Build history of the part. All positions in model axes, mm. A direction names the side the tool comes from. Coordinates: 2 decimals unless noted, no trailing zeros. Order: outer loops, then holes, each group sorted by start corner. A loop starts at its lowest first (then second) coordinate and runs counter-clockwise, first axis right, second up. Notation, with made-up numbers: (79.5, 21) - (94.5, 21) arc R27 cw to (94.5, 53) - close; hole circle Ø5 at (22, -16.5). An arc over 180 degrees is marked (long way). Write each question's results on one line, items separated by ' | '. Start each with the question number.
from build123d import *

# Parameters (mm, degrees)
EXTRUDE_1_DEPTH          = 105
SKETCH_7_W               = 30.4
SKETCH_7_H               = 19
EXTRUDE_2_DEPTH          = 3
SKETCH_8_W               = 30.4
SKETCH_8_H               = 12
EXTRUDE_3_DEPTH          = 38
FILLET_1_R               = 5
CUT_EXTRUDE_1_DEPTH      = 117
CUT_EXTRUDE_2_DEPTH      = 97
CUT_EXTRUDE_4_DEPTH      = 191.002631561
CUT_EXTRUDE_4_DEPTH_BACK = 6.8
SKETCH_11_R              = 5
FILLET_3_R               = 3
SKETCH_12_R              = 2.6
CUT_EXTRUDE_5_DEPTH      = 20
CHAMFER_1_SIZE           = 3
SKETCH_13_R              = 2.9
CUT_EXTRUDE_6_DEPTH      = 191.002631561
CHAMFER_3_SIZE           = 2.5
SKETCH_16_W              = 80
SKETCH_16_H              = 48
CUT_EXTRUDE_9_DEPTH      = 191.002631561
FILLET_4_R               = 30
SKETCH_17_W              = 28
SKETCH_17_H              = 52
CUT_EXTRUDE_10_DEPTH     = 20
FILLET_5_R               = 8
SKETCH_18_W              = 8
SKETCH_18_H              = 24
EXTRUDE_4_DEPTH          = 49
CHAMFER_4_SIZE           = 50
FILLET_6_R               = 10
SKETCH_19_R              = 2.9
CUT_EXTRUDE_11_DEPTH     = 191.002631561
CHAMFER_5_SIZE           = 2.6
SKETCH_21_R              = 2.3
CUT_EXTRUDE_13_DEPTH     = 15
FILLET_7_R               = 5
CHAMFER_6_SIZE           = 0.8
SKETCH_22_W              = 8
SKETCH_22_H              = 48.683816014
EXTRUDE_5_DEPTH          = 10
FILLET_8_R               = 10


with BuildPart() as part:
    # Sketch 2 → Extrude 1 (new body)
    with BuildSketch(Plane(origin=(0, 0, 0), x_dir=(1, 0, 0), z_dir=(0, 1, 0))):
        Polygon((52.378939236, 0), (52.378939236, -108), (24.378939236, -122), (24.378939236, -140), (0, -140), (-21.621060764, -140), (-21.621060764, 0), (-8.021060764, 0), (-8.021060764, -136), (0, -136), (22.378939236, -136), (22.378939236, 0), align=None)
    extrude(amount=EXTRUDE_1_DEPTH)



with BuildPart() as body_2:
    # Sketch 7 → Extrude 2 (new body)
    with BuildSketch(Plane.XZ):
        with Locations((7.178939236, 126.5)):
            Rectangle(SKETCH_7_W, SKETCH_7_H)
    extrude(amount=-EXTRUDE_2_DEPTH)


with BuildPart() as part_1:
    add(part.part)

    add(body_2.part)  # Extrude 3 merges body 2
    # Sketch 8 → Extrude 3 (add)
    with BuildSketch(Plane(origin=(0, 3, 0), x_dir=(1, 0, 0), z_dir=(0, 1, 0))):
        with Locations((7.178939236, -130)):
            Rectangle(SKETCH_8_W, SKETCH_8_H)
    extrude(amount=EXTRUDE_3_DEPTH)

    # Fillet 1
    fillet_1_edges = [part_1.edges().sort_by_distance(p)[0] for p in [
        (7.178939236, 41, 124),
    ]]
    fillet(fillet_1_edges, radius=FILLET_1_R)

    # Sketch 3 → Cut-Extrude 1 (cut)
    with BuildSketch(Plane(origin=(0, 0, 0), x_dir=(-1, 0, 0), z_dir=(0, 0, -1))):
        Polygon((8.021060764, -1.66), (19.321060764, 3.4), (19.321060764, 5), (8.021060764, 5), align=None)
        Polygon((-33.678939236, 5), (-22.378939236, 5), (-22.378939236, -1.66), (-33.678939236, 3.4), align=None)
    extrude(amount=-CUT_EXTRUDE_1_DEPTH, mode=Mode.SUBTRACT)

    # Sketch 9 → Cut-Extrude 2 (cut)
    with BuildSketch(Plane(origin=(0, 105, 0), x_dir=(1, 0, 0), z_dir=(0, 1, 0))):
        Polygon((-21.621060764, 0), (-21.621060764, -96), (22.378939236, -96), (22.378939236, -117), (47.378939236, -104.5), (47.378939236, 0), align=None)
    extrude(amount=-CUT_EXTRUDE_2_DEPTH, mode=Mode.SUBTRACT)

    # Sketch 11 → Cut-Extrude 4 (cut, two sides: drawn at the far end of the back side and taken through both)
    with BuildSketch(Plane.ZY.offset(21.621060764).offset(-CUT_EXTRUDE_4_DEPTH_BACK)):
        with Locations(Location((103.6, 41.2, 0), (0, 0, 180))):
            Circle(SKETCH_11_R)
    extrude(amount=CUT_EXTRUDE_4_DEPTH + CUT_EXTRUDE_4_DEPTH_BACK, mode=Mode.SUBTRACT)

    # Fillet 3
    fillet_3_edges = [part_1.edges().sort_by_distance(p)[0] for p in [
        (47.378939236, 56.5, 104.5),
        (22.378939236, 56.5, 117),
        (24.378939236, 52.5, 140),
        (24.378939236, 52.5, 122),
    ]]
    fillet(fillet_3_edges, radius=FILLET_3_R)

    # Sketch 12 → Cut-Extrude 5 (cut)
    with BuildSketch(Plane.ZY.offset(21.621060764)):
        with Locations((103.6, 41.2)):
            Circle(SKETCH_12_R)
    extrude(amount=-CUT_EXTRUDE_5_DEPTH, mode=Mode.SUBTRACT)

    # Chamfer 1
    # the kernel refuses this chamfer: 3 mm, written as the material it takes off along each edge
    with BuildSketch(Plane(origin=(-14.821060764, 41.2, 103.6), x_dir=(0, 0, 1), z_dir=(0, -1, 0))) as chamfer_1_piece_1_section:
        Polygon((2.6, -CHAMFER_1_SIZE), (2.6 + CHAMFER_1_SIZE, 0), (2.6, 0), align=None)
    chamfer_1_piece_1 = revolve(axis=Axis((-14.821060764, 41.2, 103.6), (-1, 0, 0)), mode=Mode.PRIVATE)
    chamfer_1_piece_1 = chamfer_1_piece_1 & Plane(origin=(-13.01179882, 41.2, 103.6), x_dir=(0, 0, -1), z_dir=(-1, 0, 0)) * Cylinder(5, 23, mode=Mode.PRIVATE)
    add(chamfer_1_piece_1, mode=Mode.SUBTRACT)

    # Sketch 13 → Cut-Extrude 6 (cut, through all)
    with BuildSketch(Plane.ZY.offset(21.621060764)):
        with Locations((88, 46)):
            Circle(SKETCH_13_R)
        with Locations((8, 46)):
            Circle(SKETCH_13_R)
        with Locations((88, 96)):
            Circle(SKETCH_13_R)
    extrude(amount=-CUT_EXTRUDE_6_DEPTH, mode=Mode.SUBTRACT)

    # Chamfer 3
    chamfer_3_edges = [part_1.edges().sort_by_distance(p)[0] for p in [
        (47.378939236, 96, 85.1),
        (47.378939236, 46, 5.1),
        (47.378939236, 46, 85.1),
    ]]
    chamfer(chamfer_3_edges, length=CHAMFER_3_SIZE)

    # Sketch 16 → Cut-Extrude 9 (cut, through all)
    with BuildSketch(Plane.ZY.offset(21.621060764)):
        with Locations((40, 81)):
            Rectangle(SKETCH_16_W, SKETCH_16_H)
    extrude(amount=-CUT_EXTRUDE_9_DEPTH, mode=Mode.SUBTRACT)

    # Fillet 4
    fillet_4_edges = [part_1.edges().sort_by_distance(p)[0] for p in [
        (49.878939236, 57, 80),
    ]]
    fillet(fillet_4_edges, radius=FILLET_4_R)

    # Sketch 17 → Cut-Extrude 10 (cut)
    with BuildSketch(Plane.ZY.offset(21.621060764)):
        with Locations((110, 79)):
            Rectangle(SKETCH_17_W, SKETCH_17_H)
    extrude(amount=-CUT_EXTRUDE_10_DEPTH, mode=Mode.SUBTRACT)

    # Fillet 5
    fillet_5_edges = [part_1.edges().sort_by_distance(p)[0] for p in [
        (-14.821060764, 53, 96),
        (-14.821060764, 53, 124),
    ]]
    fillet(fillet_5_edges, radius=FILLET_5_R)

    # Sketch 18 → Extrude 4 (add)
    with BuildSketch(Plane(origin=(0, 8, 0), x_dir=(1, 0, 0), z_dir=(0, 1, 0))):
        with Locations((-17.621060764, -12)):
            Rectangle(SKETCH_18_W, SKETCH_18_H)
    extrude(amount=EXTRUDE_4_DEPTH)

    # Chamfer 4
    # the kernel refuses this chamfer: 50 mm, written as the material it adds along each edge
    with BuildSketch(Plane(origin=(-13.621060764, 8, 24), x_dir=(0, 0.9996219169112966, -0.027495876610586386), z_dir=(-1, 0, 0))) as chamfer_4_piece_1_section:
        Polygon((CHAMFER_4_SIZE * 0.999621916911, -CHAMFER_4_SIZE * 0.0274958766106), (-CHAMFER_4_SIZE * 0.0274958766106, -CHAMFER_4_SIZE * 0.999621916911), (0, 0), align=None)
    chamfer_4_piece_1 = extrude(amount=8, mode=Mode.PRIVATE)
    chamfer_4_piece_1 = split(chamfer_4_piece_1, bisect_by=Plane(origin=(-17.621060764, 57, 40.555220818), z_dir=(0, -1, 0)), keep=Keep.TOP, mode=Mode.PRIVATE)
    add(chamfer_4_piece_1)

    # Fillet 6
    fillet_6_edges = [part_1.edges().sort_by_distance(p)[0] for p in [
        (49.878939236, 57, 0),
        (-17.621060764, 57, 0),
    ]]
    fillet(fillet_6_edges, radius=FILLET_6_R)

    # Sketch 19 → Cut-Extrude 11 (cut, through all)
    with BuildSketch(Plane(origin=(52.378939236, 0, 0), x_dir=(0, 0, -1), z_dir=(1, 0, 0))):
        with Locations(Location((-8, 46, 0), (0, 0, 180))):
            Circle(SKETCH_19_R)
    extrude(amount=-CUT_EXTRUDE_11_DEPTH, mode=Mode.SUBTRACT)

    # Chamfer 5
    chamfer_5_edges = [part_1.edges().sort_by_distance(p)[0] for p in [
        (-21.621060764, 46, 5.1),
    ]]
    chamfer(chamfer_5_edges, length=CHAMFER_5_SIZE)

    # Sketch 21 → Cut-Extrude 13 (cut)
    with BuildSketch(Plane.ZY.offset(21.621060764)):
        with Locations((130, 30)):
            Circle(SKETCH_21_R)
        with Locations((130, 90)):
            Circle(SKETCH_21_R)
    extrude(amount=-CUT_EXTRUDE_13_DEPTH, mode=Mode.SUBTRACT)

    # Fillet 7
    fillet_7_edges = [part_1.edges().sort_by_distance(p)[0] for p in [
        (49.878939236, 105, 80),
        (-14.821060764, 105, 124),
    ]]
    fillet(fillet_7_edges, radius=FILLET_7_R)

    # Chamfer 6
    chamfer_6_edges = [part_1.edges().sort_by_distance(p)[0] for p in [
        (-21.621060764, 41.2, 108.6),
        (-21.621060764, 30, 127.7),
        (-21.621060764, 90, 127.7),
    ]]
    chamfer(chamfer_6_edges, length=CHAMFER_6_SIZE)

    # Sketch 22 → Extrude 5 (add)
    with BuildSketch(Plane(origin=(0, 8, 0), x_dir=(1, 0, 0), z_dir=(0, 1, 0))):
        with Locations((-17.621060764, -71.658091993)):
            Rectangle(SKETCH_22_W, SKETCH_22_H)
    extrude(amount=EXTRUDE_5_DEPTH)

    # Fillet 8
    fillet_8_edges = [part_1.edges().sort_by_distance(p)[0] for p in [
        (-17.621060764, 57, 25),
    ]]
    fillet(fillet_8_edges, radius=FILLET_8_R)


solid = part_1.part
Item 1: Slice it at D-D (y = 11). Write the cut outline in (x, z), then the cut area to 3 significant figures.
Item 2: Flat gauge pins, fed straight in: P1, Ø24.5, axis at x = 10.5, y = 68, coming from the -Z side; P2, Ø3, axis at x = -12, z = 27, coming from the +Y side; P3, Ø9.5, axis at x = -17, z = 109.5, coming from the +Y side. Where does each tip first touch, or does it go through?
Item 3: Slice it at A-A (y = 96). Write the cut outline in (x, z), then the cut area to 3 significant figures.
Item 4: Slice it at C-C (z = 88). Count the separate pieces of the cut face and the enclosed holes in it, then the cut area to 3 significant figures.
Item 5: Pull direction Z, two halves, no side cores. Call faces 4 (the cylindrical face through (-17.57, 54.15, 3.01)), 5 (the flat face through (22.379, 65, 129)), 6 (the cylindrical face through (-17.57, 56.26, 24.63)): released by +Z, released by -Z, zero draft, split by the parting line, or undercut.
Item 6: Which spindle directions (+Z, -Z, +X, -X, +Y, -Y) get a long thin tool onto all of the face, cutting with end or side? Do faces 1 (the flat face through (47.379, 36, 63)), 2 (the cylindrical face through (-14.726, 50.719, 98.406)), 3 (the flat face through (29.829, 1.676, 57.681)). Say none if no direction does.
Item 7: Probe probe 1 along X at (y, z) = (13, 23.5); probe 2 along X at (y, z) = (99.5, 133.5); probe 3 along Y at (x, z) = (-10.4, 103.6). List the from-to ranges inside material, lowest first.
Item 8: Slice it at B-B (z = 44.5). Write the cut outline in (x, y), then the cut area to 3 significant figures.
Resolved:
1) outline: (-21.62, 0) - (-13.62, 0) - (-13.62, 96) - (-8.02, 96) - (-8.02, 124) - (22.38, 124) - (22.38, 118.85) arc R3 ccw to (24.04, 116.17) - (45.72, 105.33) arc R3 cw to (47.38, 102.65) - (47.38, 0) - (52.38, 0) - (52.38, 108) - (26.04, 121.17) arc R3 cw to (24.38, 123.85) - (24.38, 137) arc R3 ccw to (21.38, 140) - (-21.62, 140) - close | area: 2,580 mm^2
2) P1: z = 117.41 | P2: y = 8 | P3: y = 53
3) outline: (-21.62, 124) - (-8.02, 124) - (-8.02, 136) - (22.38, 136) - (22.38, 118.85) arc R3 ccw to (24.04, 116.17) - (45.72, 105.33) arc R3 cw to (47.38, 102.65) - (47.38, 93.4) - (49.88, 90.9) - (52.38, 90.9) - (52.38, 108) - (26.04, 121.17) arc R3 cw to (24.38, 123.85) - (24.38, 137) arc R3 ccw to (21.38, 140) - (-21.62, 140) - close; (47.38, 80) - (52.38, 80) - (52.38, 85.1) - (49.88, 85.1) - (47.38, 82.6) - close | area: 634 mm^2
4) separate pieces: 4 | enclosed holes: 0 | area: 756 mm^2
5) face 4: released by -Z | face 5: zero draft | face 6: undercut
6) face 1: -Z, +Y | face 2: -X, +Y | face 3: -Z
7) probe 1: -21.62 to -13.62, 47.38 to 52.38 | probe 2: -21.62 to -8.02, 22.38 to 24.38 | probe 3: 5 to 38.6, 43.8 to 52.99
8) outline: (-21.62, 0) - (-11.73, 0) - (-19.32, 3.4) - (-19.32, 5) - (-8.02, 5) - (-8.02, 8) - (-13.62, 8) - (-13.62, 37.5) - (-21.62, 37.5) - close; (22.38, 5) - (33.68, 5) - (33.68, 3.4) - (26.09, 0) - (52.38, 0) - (52.38, 57) - (47.38, 57) - (47.38, 8) - (22.38, 8) - close | area: 743 mm^2
